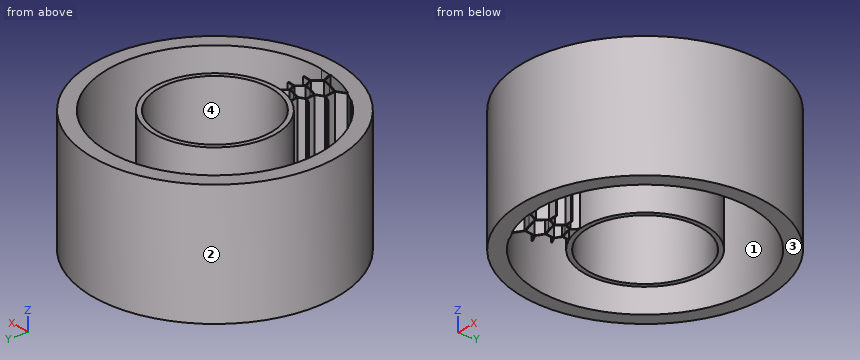
```python
from build123d import *

# Parameters (mm, degrees)
BOSS_EXTRUDE1_DEPTH = 40
SKETCH1_6_R         = 40
SKETCH1_6_R_2       = 35
SKETCH1_6_R_3       = 20
SKETCH1_6_R_4       = 18.5
BOSS_EXTRUDE2_DEPTH = 40


with BuildPart() as part:
    # Sketch1 → Boss-Extrude1 (new body)
    with BuildSketch(Plane.XY):
        with BuildLine():
            Line((0, -29.2), (0, -29))
            Line((0, -29), (-2.896372732, -28.855))
            Line((-2.896372732, -28.855), (-5.153701873, -31.582263329))
            Line((-5.153701873, -31.582263329), (-3.495622262, -34.825))
            ThreePointArc((-3.495622262, -34.825), (-1.75, -34.956222622), (0, -35))
            Line((0, -35), (0, -34.8))
            Line((0, -34.8), (-3.370043386, -34.631286807))
            Line((-3.370043386, -34.631286807), (-4.915711127, -31.608396089))
            Line((-4.915711127, -31.608396089), (-2.806033523, -29.059522617))
            Line((-2.806033523, -29.059522617), (0, -29.2))
        make_face()
        with BuildLine():
            Line((-3.495622262, -34.825), (-5.153701873, -31.582263329))
            Line((-5.153701873, -31.582263329), (-8.282209443, -30.909626441))
            Line((-8.282209443, -30.909626441), (-8.334038079, -31.103053542))
            Line((-8.334038079, -31.103053542), (-5.288554278, -31.757840113))
            Line((-5.288554278, -31.757840113), (-3.732843691, -34.800371808))
            ThreePointArc((-3.732843691, -34.800371808), (-3.614253954, -34.812887963), (-3.495622262, -34.825))
        make_face()
        Polygon((-5.153701873, -31.582263329), (-2.896372732, -28.855), (-4.278593468, -26.219534795), (-6.875874487, -25.661112933), (-6.927703123, -25.854540034), (-4.412206949, -26.395377951), (-3.135314054, -28.830015709), (-5.230359841, -31.36121129), (-8.230380808, -30.716199341), (-8.282209443, -30.909626441), align=None)
        Polygon((-2.896372732, -28.855), (0, -29), (0, -28.8), (-2.772167607, -28.661218034), (-4.040561936, -26.2427844), (-2.303365501, -24.084687494), (0, -24.2), (0, -24), (-2.395409567, -23.880079527), (-4.278593468, -26.219534795), align=None)
        Polygon((-6.875874487, -25.661112933), (-4.278593468, -26.219534795), (-2.395409567, -23.880079527), (-3.543170038, -21.712806039), (-5.694018992, -21.250368178), (-5.745847628, -21.443795279), (-3.676306485, -21.888751758), (-2.633800725, -23.857276683), (-4.357083522, -25.998088853), (-6.824045852, -25.467685833), align=None)
        with BuildLine():
            Line((-3.543170038, -21.712806039), (-2.395409567, -23.880079527))
            Line((-2.395409567, -23.880079527), (0, -24))
            Line((0, -24), (0, -23.8))
            Line((0, -23.8), (-2.271732982, -23.686271101))
            Line((-2.271732982, -23.686271101), (-3.30286447, -21.73922379))
            Line((-3.30286447, -21.73922379), (-1.754210625, -19.922920094))
            ThreePointArc((-1.754210625, -19.922920094), (-1.875889536, -19.91183162), (-1.997498436, -19.9))
            Line((-1.997498436, -19.9), (-3.543170038, -21.712806039))
        make_face()
        with BuildLine():
            Line((-5.694018992, -21.250368178), (-3.543170038, -21.712806039))
            Line((-3.543170038, -21.712806039), (-1.997498436, -19.9))
            ThreePointArc((-1.997498436, -19.9), (-2.118012645, -19.887534348), (-2.238449128, -19.874338869))
            Line((-2.238449128, -19.874338869), (-3.617879715, -21.492172887))
            Line((-3.617879715, -21.492172887), (-5.642190357, -21.056941078))
            Line((-5.642190357, -21.056941078), (-5.694018992, -21.250368178))
        make_face()
    boss_extrude1 = extrude(amount=BOSS_EXTRUDE1_DEPTH)

    # Sketch1<6> → Boss-Extrude2 (add)
    with BuildSketch(Plane.XY):
        Circle(SKETCH1_6_R)
        Circle(SKETCH1_6_R_2, mode=Mode.SUBTRACT)
        Circle(SKETCH1_6_R_3)
        Circle(SKETCH1_6_R_4, mode=Mode.SUBTRACT)
    extrude(amount=BOSS_EXTRUDE2_DEPTH)

    # Mirror1: Boss-Extrude1 across plane
    add(boss_extrude1.mirror(Plane(origin=(0, 0, 40), x_dir=(0, 0, 1), z_dir=(0.9659258262890685, -0.2588190451025203, 0))))


solid = part.part
```
The model under review builds one solid part; all positions refer to its coordinate system, in mm. Face numbers are marked on the shaded views. Round coordinates to 2 decimals unless told otherwise and drop trailing zeros. Loops run counter-clockwise (first coordinate to the right, second up) from the corner with the lowest first, then second, coordinate; pieces in that order, holes last. Notation, with made-up numbers: M 84.25,73.5 L 109.25,73.5 A20 ccw 109.25,96.5 Z; hole C 23,-26.75 d8. An arc over 180 degrees is marked long. Write item = value, one per line.
Item 1: For line 1 (X direction, y = 1.5, z = 18); line 2 (X direction, y = 11, z = 15); line 3 (Y direction, x = -22, z = 23.5), list the stretches that pass through material, from the lowest coordinate up. Write a range as [from, to].
Return value:
line_1 = [-39.97, -34.97], [-19.94, -18.44], [18.44, 19.94], [34.97, 39.97]
line_2 = [-38.46, -33.23], [-16.7, -14.87], [14.87, 16.7], [33.23, 38.46]
line_3 = [-33.41, -27.22], [27.22, 33.41]
Item 2: Take a section at C-C on y = 22. Write out the cut boundary in (x, z).
Return value:
outline = M -33.41,0 L -27.22,0 L -27.22,40 L -33.41,40 Z; M 27.22,0 L 33.41,0 L 33.41,40 L 27.22,40 Z
Item 3: Take a section at B-B on x = 5. Write out the cut boundary in (y, z), then the cut area to 3 significant figures.
Return value:
outline = M -39.69,0 L -34.64,0 L -34.64,40 L -39.69,40 Z; M -19.36,0 L -17.81,0 L -17.81,40 L -19.36,40 Z; M 17.81,0 L 19.36,0 L 19.36,40 L 17.81,40 Z; M 34.64,0 L 39.69,0 L 39.69,40 L 34.64,40 Z
area = 528 mm2
Item 4: The part is to be moulded in two halves that separate along Y. For the marked faces 1, 2, 3 and 4, say which applies: released by +Y, released by -Y, zero draft, split by the parting line, or undercut.
Return value:
face_1 = undercut
face_2 = split by the parting line
face_3 = zero draft
face_4 = undercut
Item 5: Take a section at D-D on z = 31. State how many separate pieces and enclosed holes the cut face has, then the cut area to 3 significant figures.
Return value:
separate_pieces = 1
enclosed_holes = 6
area = 1,390 mm2
Item 6: Insertion check: P1, Ø2, axis at x = -8, z = 11.5, coming from the -Y side; P2, Ø1, axis at y = 6, z = 14.5, coming from the +X side; P3, Ø1.5, axis at y = 2.5, z = 21.5, coming from the +X side; P4, Ø12, axis at x = -9, y = 27.5, coming from the +Z side. Each pin has a flat end and moves straight along its axis. Give the tip position at first contact, or say it passes through.
Return value:
P1 = -39.38
P2 = 39.62
P3 = 39.96
P4 = through
Item 7: Take a section at A-A on y = 0. Write out the cut boundary in (x, z), then the cut area to 3 significant figures.
Return value:
outline = M -40,0 L -35,0 L -35,40 L -40,40 Z; M -20,0 L -18.5,0 L -18.5,40 L -20,40 Z; M 18.5,0 L 20,0 L 20,40 L 18.5,40 Z; M 35,0 L 40,0 L 40,40 L 35,40 Z
area = 520 mm2
